The listing builds one solid part. Answer for the finished solid, in the listing's coordinates (mm). Face numbers are marked on the shaded views. A direction names the side the tool comes from. Coordinates: 2 decimals unless noted, no trailing zeros. Order: outer loops, then holes, each group sorted by start corner. A loop starts at its lowest first (then second) coordinate and runs counter-clockwise, first axis right, second up.
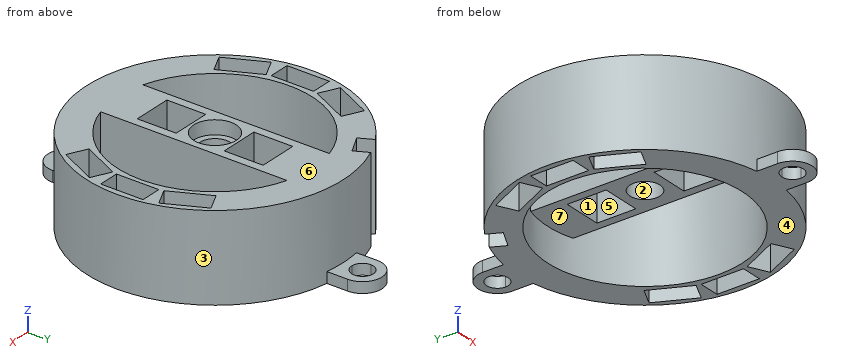
```python
from build123d import *

# Parameters (mm, degrees)
SKETCH1_R                       = 29.64
SKETCH1_R_2                     = 22.5
BOSS_EXTRUDE1_DEPTH             = 19.92
SKETCH4_W                       = 12.873355566
SKETCH4_H                       = 48.428243032
BOSS_EXTRUDE3_DEPTH             = 3.175
CUT_EXTRUDE2_REACH              = 48.41
SKETCH7_R                       = 4.9125
CUT_EXTRUDE2_DIRECTION_2_DEPTH  = 47.409757595
SKETCH8_W                       = 12.873355566
SKETCH8_H                       = 48.17275248
SKETCH8_R                       = 3.475
BOSS_EXTRUDE4_DEPTH             = 9
SKETCH1_3_W                     = 4.8
SKETCH1_3_H                     = 9.8
CUT_EXTRUDE1_DEPTH              = 20
CIRPATTERN1_COUNT               = 2
CIRPATTERN1_ANGLE               = 26
CIRPATTERN1_THE_OTHER_WAY_COUNT = 2
CIRPATTERN1_THE_OTHER_WAY_ANGLE = 26
SKETCH11_W                      = 9
SKETCH11_H                      = 9
CUT_EXTRUDE21_DEPTH             = 29
BOSS_EXTRUDE5_DEPTH             = 2.5
MIRROR3_COPY_1_SKETCH_W         = 4.8
MIRROR3_COPY_1_SKETCH_H         = 9.8
MIRROR3_COPY_1_DEPTH            = 20
MIRROR3_COPY_2_SKETCH_W         = 4.8
MIRROR3_COPY_2_SKETCH_H         = 9.8
MIRROR3_COPY_2_DEPTH            = 20
CUT_EXTRUDE22_DEPTH             = 53.615450202
CUT_EXTRUDE22_DEPTH_BACK        = 53.615450202


with BuildPart() as part:
    # Sketch1 → Boss-Extrude1 (new body)
    with BuildSketch(Plane.XY):
        Circle(SKETCH1_R)
        Circle(SKETCH1_R_2, mode=Mode.SUBTRACT)
    extrude(amount=BOSS_EXTRUDE1_DEPTH)

    # Sketch4 → Boss-Extrude3 (add)
    with BuildSketch(Plane.XY.offset(19.92)):
        Rectangle(SKETCH4_W, SKETCH4_H)
    extrude(amount=-BOSS_EXTRUDE3_DEPTH)

    # Sketch7 → Cut-Extrude2 (cut, up to next)
    with BuildSketch(Plane.XY.offset(19.92), mode=Mode.PRIVATE) as cut_extrude2_sk1:
        with Locations(Location((0, 0, 0), (0, 0, 180))):
            Circle(SKETCH7_R)
    cut_extrude2_tool1 = extrude(cut_extrude2_sk1.sketch, amount=-CUT_EXTRUDE2_REACH, mode=Mode.PRIVATE) & part.part
    add(cut_extrude2_tool1.solids().sort_by_distance((0, 0, 19.92))[0], mode=Mode.SUBTRACT)

    # Sketch7 → Cut-Extrude2 direction 2 (cut)
    with BuildSketch(Plane.XY.offset(19.92)):
        with Locations(Location((0, 0, 0), (0, 0, 180))):
            Circle(SKETCH7_R)
    extrude(amount=CUT_EXTRUDE2_DIRECTION_2_DEPTH, mode=Mode.SUBTRACT)

    # Sketch8 → Boss-Extrude4 (add)
    with BuildSketch(Plane.XY.offset(16.745)):
        Rectangle(SKETCH8_W, SKETCH8_H)
        Circle(SKETCH8_R, mode=Mode.SUBTRACT)
    extrude(amount=-BOSS_EXTRUDE4_DEPTH)

    # Sketch1<3> → Cut-Extrude1 (cut)
    with BuildSketch(Plane.XY):
        with Locations((25.9, 0)):
            Rectangle(SKETCH1_3_W, SKETCH1_3_H)
    cut_extrude1 = extrude(amount=CUT_EXTRUDE1_DEPTH, mode=Mode.SUBTRACT)

    # CirPattern1: Cut-Extrude1 ×2 about axis
    cirpattern1_axis = Axis((0, 0, 0), (0, 0, 1))
    for i in range(1, CIRPATTERN1_COUNT):
        add(cut_extrude1.rotate(cirpattern1_axis, i * CIRPATTERN1_ANGLE / (CIRPATTERN1_COUNT - 1)), mode=Mode.SUBTRACT)

    # CirPattern1 the other way: Cut-Extrude1 ×2 about axis
    cirpattern1_the_other_way_axis = Axis((0, 0, 0), (0, 0, -1))
    for i in range(1, CIRPATTERN1_THE_OTHER_WAY_COUNT):
        add(cut_extrude1.rotate(cirpattern1_the_other_way_axis, i * CIRPATTERN1_THE_OTHER_WAY_ANGLE / (CIRPATTERN1_THE_OTHER_WAY_COUNT - 1)), mode=Mode.SUBTRACT)

    # Sketch11 → Cut-Extrude21 (cut)
    with BuildSketch(Plane(origin=(0, 0, 19.92), x_dir=(-1, 0, 0), z_dir=(0, 0, -1))):
        with Locations((0, 10.0625)):
            Rectangle(SKETCH11_W, SKETCH11_H)
    cut_extrude21 = extrude(amount=CUT_EXTRUDE21_DEPTH, mode=Mode.SUBTRACT)

    # Mirror1: Cut-Extrude21 across plane
    add(cut_extrude21.mirror(Plane.ZX), mode=Mode.SUBTRACT)

    # Sketch12 → Boss-Extrude5 (add)
    with BuildSketch(Plane(origin=(0, 0, 0), x_dir=(-1, 0, 0), z_dir=(0, 0, -1))):
        with BuildLine():
            Line((0, 29.64), (0, 31.64))
            ThreePointArc((0, 31.64), (-1.767766953, 32.372233047), (-2.5, 34.14))
            Line((-2.5, 34.14), (-4.5, 34.14))
            Line((-4.5, 34.14), (-4.5, 29.296409336))
            ThreePointArc((-4.5, 29.296409336), (-2.256549055, 29.553977505), (0, 29.64))
        make_face()
        with BuildLine():
            ThreePointArc((2.5, 34.14), (1.767766953, 32.372233047), (0, 31.64))
            Line((0, 31.64), (0, 29.64))
            ThreePointArc((0, 29.64), (2.256549055, 29.553977505), (4.5, 29.296409336))
            Line((4.5, 29.296409336), (4.5, 34.14))
            ThreePointArc((4.5, 34.14), (0, 38.64), (-4.5, 34.14))
            Line((-4.5, 34.14), (-2.5, 34.14))
            ThreePointArc((-2.5, 34.14), (0, 36.64), (2.5, 34.14))
        make_face()
    boss_extrude5 = extrude(amount=-BOSS_EXTRUDE5_DEPTH)

    # Mirror2: Boss-Extrude5 across plane
    add(boss_extrude5.mirror(Plane.ZX))

    # Mirror3: Cut-Extrude1 across plane
    add(cut_extrude1.mirror(Plane(origin=(0, 0, 0), x_dir=(0, 0, 1), z_dir=(1, 0, 0))), mode=Mode.SUBTRACT)

    # Mirror3 copy 1 sketch → Mirror3 copy 1 (cut)
    with BuildSketch(Plane(origin=(0, 0, 0), x_dir=(-0.8987940462991663, 0.43837114678907885, 0), z_dir=(0, 0, 1))):
        with Locations((25.9, 0)):
            Rectangle(MIRROR3_COPY_1_SKETCH_W, MIRROR3_COPY_1_SKETCH_H)
    extrude(amount=MIRROR3_COPY_1_DEPTH, mode=Mode.SUBTRACT)

    # Mirror3 copy 2 sketch → Mirror3 copy 2 (cut)
    with BuildSketch(Plane(origin=(0, 0, 0), x_dir=(-0.8987940462991663, -0.43837114678907885, 0), z_dir=(0, 0, 1))):
        with Locations((25.9, 0)):
            Rectangle(MIRROR3_COPY_2_SKETCH_W, MIRROR3_COPY_2_SKETCH_H)
    extrude(amount=MIRROR3_COPY_2_DEPTH, mode=Mode.SUBTRACT)

    # Sketch13 → Cut-Extrude22 (cut, two sides: drawn at the far end of the back side and taken through both)
    with BuildSketch(Plane.XY.offset(-CUT_EXTRUDE22_DEPTH_BACK)):
        Polygon((-9.760082808, 24.264783614), (-14.199291993, 21.964039863), (-15.809812619, 25.071486294), (-11.370603433, 27.372230044), align=None)
        Polygon((-16.779237208, 26.941959066), (-12.340028022, 29.242702816), (-11.370603433, 27.372230044), (-15.809812619, 25.071486294), align=None)
    extrude(amount=CUT_EXTRUDE22_DEPTH + CUT_EXTRUDE22_DEPTH_BACK, mode=Mode.SUBTRACT)


solid = part.part
```
(1) Find section A-A (y = 0). Write down the section's boundary in (x, z) (1 decimal).
(2) The mould has two halves that part along X. Classify the marked faces 1, 2, 3 and 4: released by +X, released by -X, zero draft, split by the parting line, or undercut.
(3) Consider line 1 (Y direction, x = 0, z = 18.7); line 2 (Y direction, x = 0, z = 12.25) (1 decimal); line 3 (Y direction, x = 0, z = 4.75). Determine where each line is inside the solid, lowest interval first.
(4) Find section D-D (x = 21). Write down the section's boundary in (y, z).
(5) Find section B-B (x = 15). Write down the section's boundary in (y, z), and give its area (3 significant figures).
(6) Each of these flat-tipped pins is pushed along its axis until it touches: pin 1 Ø7 at (x, z) = (-1, 11.5) entering from +Y; pin 2 Ø2.5 at (x, z) = (25, 5) entering from +Y; pin 3 Ø4.5 at (x, y) = (1, 34) entering from +Z. Where does it stop, or does it pass through?
(7) For the marked faces 5, 6 and 7, determine the directions among +Z, -Z, +X, -X, +Y, -Y from which every point of the face is accessible in a straight line to the end or side of a thin tool.
(8) Find section C-C (y = 16). Write down the section's boundary in (x, z) (3 decimals), and give its area (3 significant figures).
Findings below:
1. outline: (-29.6, 0) - (-28.3, 0) - (-28.3, 19.9) - (-29.6, 19.9) - close; (-23.5, 0) - (-22.5, 0) - (-22.5, 19.9) - (-23.5, 19.9) - close; (-6.4, 7.7) - (-3.5, 7.7) - (-3.5, 16.7) - (-4.9, 16.7) - (-4.9, 19.9) - (-6.4, 19.9) - close; (3.5, 7.7) - (6.4, 7.7) - (6.4, 19.9) - (4.9, 19.9) - (4.9, 16.7) - (3.5, 16.7) - close; (22.5, 0) - (23.5, 0) - (23.5, 19.9) - (22.5, 19.9) - close; (28.3, 0) - (29.6, 0) - (29.6, 19.9) - (28.3, 19.9) - close
2. face 1: undercut
2. face 2: undercut
2. face 3: split by the parting line
2. face 4: zero draft
3. line 1: y = -29.64 to -14.56, -5.56 to -4.91, 4.91 to 5.56, 14.56 to 29.64
3. line 2: y = -29.6 to -14.6, -5.6 to -3.5, 3.5 to 5.6, 14.6 to 29.6
3. line 3: y = -29.64 to -22.5, 22.5 to 29.64
4. outline: (-20.92, 0) - (-15.69, 0) - (-15.69, 19.92) - (-20.92, 19.92) - close; (-10.55, 0) - (-8.08, 0) - (-8.08, 19.92) - (-10.55, 19.92) - close; (8.08, 0) - (10.55, 0) - (10.55, 19.92) - (8.08, 19.92) - close; (15.69, 0) - (20.92, 0) - (20.92, 19.92) - (15.69, 19.92) - close
5. outline: (-25.56, 0) - (-16.77, 0) - (-16.77, 19.92) - (-25.56, 19.92) - close; (16.77, 0) - (25.56, 0) - (25.56, 19.92) - (16.77, 19.92) - close
5. area: 350 mm2
6. pin 1: stops at y = 29.64
6. pin 2: stops at y = 17.73
6. pin 3: stops at z = 2.5
7. face 5: +Z, -Z
7. face 6: +Z, +X, -X, +Y, -Y
7. face 7: -Z
8. outline: (-24.951, 0) - (-23.683, 0) - (-23.683, 19.92) - (-24.951, 19.92) - close; (-21.627, 0) - (-15.819, 0) - (-15.819, 19.92) - (-21.627, 19.92) - close; (-6.437, 7.745) - (6.437, 7.745) - (6.437, 19.92) - (-6.437, 19.92) - close; (15.819, 0) - (21.627, 0) - (21.627, 19.92) - (15.819, 19.92) - close; (23.683, 0) - (24.951, 0) - (24.951, 19.92) - (23.683, 19.92) - close
8. area: 439 mm2
